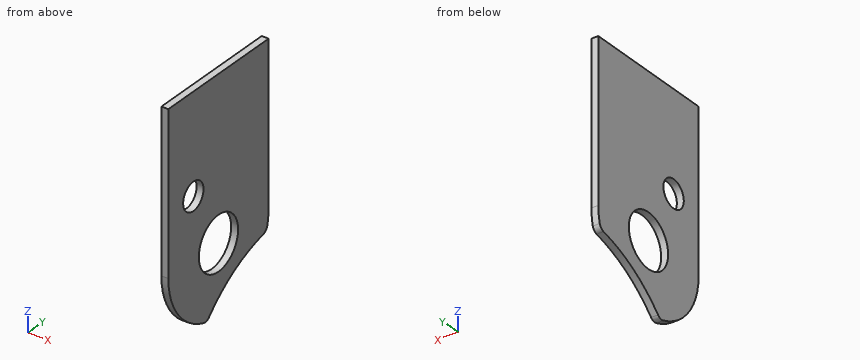
from build123d import *

# Parameters (mm, degrees)
SKETCH1_R               = 9.65
BASE_FLANGE1_DEPTH      = 2.5
CUT_EXTRUDE1_DEPTH      = 63.525520722
CUT_EXTRUDE1_DEPTH_BACK = 63.525520722
SKETCH2_R               = 5
SKETCH2_R_2             = 52.175
FILLET1_R               = 2.5
SCALE1_SCALE            = 1.5


# Sheet-metal steps are written as plain solids
with BuildPart() as part:
    # Sketch1 → Base-Flange1 (new body)
    with BuildSketch(Plane(origin=(0, 0, 0), x_dir=(0, 0, -1), z_dir=(1, 0, 0))):
        with BuildLine():
            Line((0, 24.65), (-57.40704, 24.65))
            Line((-57.40704, 24.65), (-57.40704, -24.65))
            Line((-57.40704, -24.65), (0, -24.65))
            ThreePointArc((0, -24.65), (24.65, 0), (0, 24.65))
        make_face()
        Circle(SKETCH1_R, mode=Mode.SUBTRACT)
    extrude(amount=-BASE_FLANGE1_DEPTH)

    # Sketch2 → Cut-Extrude1 (cut, two sides: drawn at the far end of the back side and taken through both)
    with BuildSketch(Plane(origin=(0, 0, 0), x_dir=(0, 0, -1), z_dir=(1, 0, 0)).offset(-CUT_EXTRUDE1_DEPTH_BACK)):
        with Locations((-21.8797706, -12.3562513)):
            Circle(SKETCH2_R)
        with Locations((58.59296, 33.3400694)):
            Circle(SKETCH2_R_2)
    extrude(amount=CUT_EXTRUDE1_DEPTH + CUT_EXTRUDE1_DEPTH_BACK, mode=Mode.SUBTRACT)

    # Fillet1
    fillet1_edges = [part.edges().sort_by_distance(p)[0] for p in [
        (-1.25, 23.529116974, -7.348683856),
        (-1.25, -5.701899087, -23.981468821),
    ]]
    fillet(fillet1_edges, radius=FILLET1_R)


with BuildPart() as part_1:
    # Scale1: scaled about (-1.25, -0.353186923, 22.904210984)
    add(part.part.scale(SCALE1_SCALE).moved(Location((0.625, 0.176593461, -11.452105492))))


solid = part_1.part
The listing builds one solid part. Answer for the finished solid, in the listing's coordinates (mm). Give positions to 0.01 mm unless a question says otherwise; leave off trailing zeros. Write each loop counter-clockwise with the first axis right and the second up, starting at its lowest first coordinate (ties: lowest second). Pieces come first, ordered by that corner, then holes.
Item 1: Section C-C, the plane x = -2.55 is taken. Count the separate pieces of the cut face and the enclosed holes in it, plus the area to 3 significant figures.
Item 2: Section B-B, the plane y = 11 is taken. Write down the section's boundary in (x, z) (3 decimals).
Item 3: Section A-A, the plane z = 0 is taken. Write down the section's boundary in (x, y) (3 decimals).
Item 4: Find the intervals of material crossed by line 1 along Z through (x, y) = (0.3, -11.5); line 2 along Y through (x, z) = (0.1, -12); line 3 along Y through (x, z) = (-0.55, -16), in increasing order.
Item 5: Section D-D, the plane y = 27 is taken. Write down the section's boundary in (x, z) (3 decimals).
Completed:
1. separate pieces: 1
1. enclosed holes: 2
1. area: 7,190 mm2
2. outline: (-3.125, -31.596) - (0.625, -31.596) - (0.625, -21.064) - (-3.125, -21.064) - close; (-3.125, -1.841) - (0.625, -1.841) - (0.625, 74.658) - (-3.125, 74.658) - close
3. outline: (-3.125, -36.798) - (0.625, -36.798) - (0.625, -8.676) - (-3.125, -8.676) - close; (-3.125, 9.03) - (0.625, 9.03) - (0.625, 37.152) - (-3.125, 37.152) - close
4. line 1: z = -46.53 to -20.01, -2.9 to 18.33, 24.4 to 74.66
4. line 2: y = -36.79 to -14.29, 14.64 to 37.15
4. line 3: y = -36.52 to -13.57, 13.92 to 36.87
5. outline: (-3.125, -24.593) - (0.625, -24.593) - (0.625, 74.658) - (-3.125, 74.658) - close
